from build123d import *

# Parameters (mm, degrees)
SKETCH1_W           = 35.5
SKETCH1_H           = 75.5
BOSS_EXTRUDE1_DEPTH = 1.5
BOSS_EXTRUDE2_DEPTH = 1.5
SKETCH2_R           = 11
CUT_EXTRUDE1_DEPTH  = 10
CUT_EXTRUDE2_DEPTH  = 2.5
SKETCH4_R           = 1.9
CUT_EXTRUDE3_DEPTH  = 6
FILLET1_R           = 0.5
FILLET2_R           = 0.5
FILLET3_R           = 1


with BuildPart() as part:
    # Sketch1 → Boss-Extrude1 (new body)
    with BuildSketch(Plane(origin=(0, 0, 0), x_dir=(1, 0, 0), z_dir=(0, 1, 0))):
        with Locations((17.75, 37.75)):
            Rectangle(SKETCH1_W, SKETCH1_H)
    extrude(amount=BOSS_EXTRUDE1_DEPTH)

    # 3DSketch1 → Boss-Extrude2 (add)
    with BuildSketch(Plane(origin=(1.85, 1.5, -1.85), x_dir=(0.40495657653791334, 0, -0.9143359180950364), z_dir=(0, 1, 0))):
        Polygon((0, 0), (12.877619134, -29.075882195), (78.526938053, 0), (65.649318919, 29.075882195), align=None)
    extrude(amount=BOSS_EXTRUDE2_DEPTH)

    # Sketch2 → Cut-Extrude1 (cut)
    with BuildSketch(Plane(origin=(0, 3, 0), x_dir=(1, 0, 0), z_dir=(0, 1, 0))):
        with Locations(Location((17.75, 18.6, 0), (0, 0, 270))):
            Circle(SKETCH2_R)
    extrude(amount=-CUT_EXTRUDE1_DEPTH, mode=Mode.SUBTRACT)

    # 3DSketch2 → Cut-Extrude2 (cut)
    with BuildSketch(Plane(origin=(17.75, 3, -6.3), x_dir=(-0.004227803372085647, 0, -0.9999910627993868), z_dir=(0, -1, 0))):
        with BuildLine():
            add(Edge.make_bspline(
                [(0, 0), (0.004386995, -1.04174525), (0.27944755, -3.123987084), (1.476453938, -6.075565296), (3.410311469, -8.653144172), (5.973707785, -10.661776555), (8.970625928, -11.936313966), (12.195586401, -12.389659387), (15.427695721, -11.99044335), (18.445556685, -10.766344357), (21.042285232, -8.800917271), (23.040178447, -6.229084123), (24.302092158, -3.226838845), (24.741880785, 0), (24.329080551, 3.230402285), (23.092306587, 6.243090971), (21.115981025, 8.831534564), (18.535772158, 10.818599013), (15.528248734, 12.067881173), (12.299589709, 12.494101301), (9.070951129, 12.06772549), (6.063488405, 10.818297059), (3.483374022, 8.831111933), (1.507182222, 6.242560327), (0.270527087, 3.229871892), (-0.004531746, 1.07611808), (0, 0)],
                knots=[0, 0, 0, 0, 0.04044329, 0.080893626, 0.122671197, 0.164448751, 0.206226312, 0.248003874, 0.289781435, 0.331558997, 0.373336558, 0.415114119, 0.456891681, 0.498669242, 0.540446803, 0.582224365, 0.624001926, 0.665779488, 0.707557049, 0.74933461, 0.791112172, 0.832889733, 0.874667296, 0.916444855, 0.958222266, 1, 1, 1, 1], degree=3))
        make_face()
    extrude(amount=CUT_EXTRUDE2_DEPTH, mode=Mode.SUBTRACT)

    # Sketch4 → Cut-Extrude3 (cut)
    with BuildSketch(Plane(origin=(0, 3, 0), x_dir=(1, 0, 0), z_dir=(0, 1, 0))):
        with Locations(Location((12.975, 63.925, 0), (0, 0, 270))):
            Circle(SKETCH4_R)
    extrude(amount=-CUT_EXTRUDE3_DEPTH, mode=Mode.SUBTRACT)

    # Fillet1
    fillet1_edges = [part.edges().sort_by_distance(p)[0] for p in [
        (12.975, 3, -65.825),
    ]]
    fillet(fillet1_edges, radius=FILLET1_R)

    # Fillet2
    fillet2_edges = [part.edges().sort_by_distance(p)[0] for p in [
        (12.975, 0, -65.825),
    ]]
    fillet(fillet2_edges, radius=FILLET2_R)

    # Fillet3
    fillet3_edges = [part.edges().sort_by_distance(p)[0] for p in [
        (17.749997791, 3, -30.899997542),
    ]]
    fillet(fillet3_edges, radius=FILLET3_R)


solid = part.part
Read the model definition and answer for the solid it produces. Units are mm, in the model's axes. A direction names the side the tool comes from. Round coordinates to 2 decimals unless told otherwise and drop trailing zeros.
Q1. Each of these flat-tipped pins is pushed along its axis until it touches: pin 1 (7.5 mm diameter, centred on x = 21.5, z = -14.5, fed in from +Y); pin 2 (1.2 mm diameter, centred on y = 2.5, z = -51.5, fed in from -X). Where does it stop, or does it pass through?
Q2. Which of the six approach directions +Z, -Z, +X, -X, +Y, -Y give full straight-line access (tool end or side, diameter ignored) to faces 1 (the face through (33.65, 2, -37)), 2 (the face through (1, 1.5, -38)), 3 (the face through (1.85, 2, -38))?
Q3. Consider probe 1 along Z at (x, y) = (14, 2.7); probe 2 along Z at (x, y) = (21.5, 0.45); probe 3 along X at (y, z) = (0.1, -18.6). Determine where each line is inside the solid, lowest interval first.
Output:
1. pin 1: passes through
1. pin 2: stops at x = 1.85
2. face 1: +Z, -Z, +X, +Y
2. face 2: +Y
2. face 3: +Z, -Z, -X, +Y
3. probe 1: z = -73.65 to -65.57, -62.28 to -30.61, -6.59 to -1.85
3. probe 2: z = -75.5 to -28.94, -8.26 to 0
3. probe 3: x = 0 to 6.75, 28.75 to 35.5
